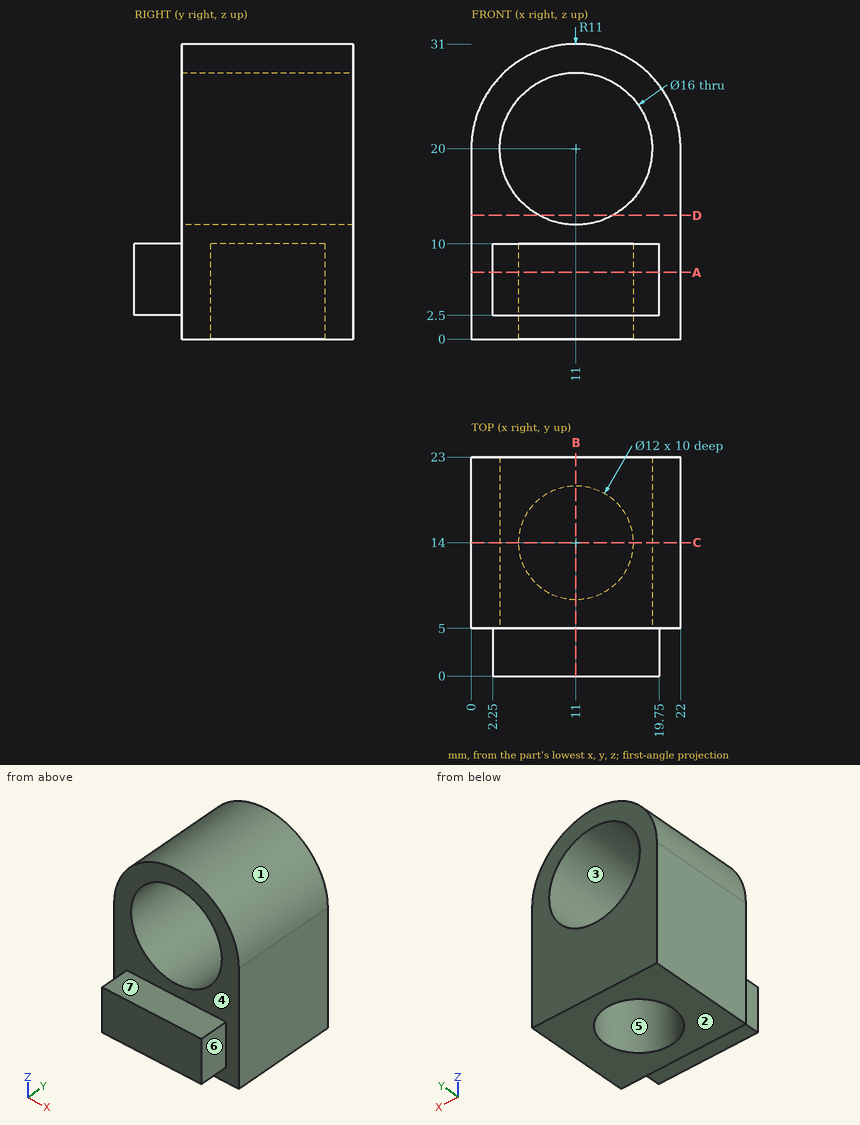
Input: dimensioned drawing with shaded views. Units: mm. Origin: part minimum x, y, z. A direction names the side the tool comes from. Coordinates: 2 decimals unless noted, no trailing zeros. Order: outer loops, then holes, each group sorted by start corner. A loop starts at its lowest first (then second) coordinate and runs counter-clockwise, first axis right, second up.
(1) Material intervals for probe 1 along Y at (x, z) = (11, 6.75); probe 2 along X at (y, z) = (17.75, 20); probe 3 along Z at (x, y) = (10, 2.5), sorted ascending.
(2) Section query C-C (y = 14). Return the cut outline in (x, z), plus the area to 3 significant figures.
(3) Draft query along Z for the marked faces 1, 2, 3 and 4. Return one class per face: pulls with the +Z half, pulls with the -Z half, needs draft (parallel to the pull), parting line crosses it, or undercut.
(4) Section query D-D (z = 13). Return the cut outline in (x, y).
(5) Access query for the marked faces 5, 6 and 7. Directions: +Z, -Z, +X, -X, +Y, -Y. A direction counts if a zero-diameter tool reaches every point of the face in a straight line with its end or side. Return the directions, or none.
(6) First-contact query: pin 1 (4 mm diameter, centred on x = 14, y = 2, fed in from -Z); pin 2 (2.5 mm diameter, centred on y = 2, z = 8, fed in from -X); pin 3 (1 mm diameter, centred on x = 19, y = 18.5, fed in from +Z). Flat tips, straight axial feed; report the tip coordinate or a pass-through.
(7) Section query A-A (z = 7). Return the cut outline in (x, y), plus the area to 3 significant figures.
(8) Section query B-B (x = 11). Return the cut outline in (y, z).
Solution:
1. probe 1: y = 0 to 8, 20 to 23
1. probe 2: x = 0 to 3, 19 to 22
1. probe 3: z = 2.5 to 10
2. outline: (0, 0) - (5, 0) - (5, 10) - (17, 10) - (17, 0) - (22, 0) - (22, 20) arc R11 ccw to (0, 20) - close; hole circle Ø16 at (11, 20)
2. area: 309 mm2
3. face 1: pulls with the +Z half
3. face 2: pulls with the -Z half
3. face 3: undercut
3. face 4: needs draft
4. outline: (0, 5) - (7.13, 5) - (7.13, 23) - (0, 23) - close; (14.87, 5) - (22, 5) - (22, 23) - (14.87, 23) - close
5. face 5: -Z
5. face 6: +Z, -Z, +X, -Y
5. face 7: +Z, +X, -X, -Y
6. pin 1: stops at z = 2.5
6. pin 2: stops at x = 2.25
6. pin 3: stops at z = 28.05
7. outline: (0, 5) - (2.25, 5) - (2.25, 0) - (19.75, 0) - (19.75, 5) - (22, 5) - (22, 23) - (0, 23) - close; hole circle Ø12 at (11, 14)
7. area: 370 mm2
8. outline: (0, 2.5) - (5, 2.5) - (5, 0) - (8, 0) - (8, 10) - (20, 10) - (20, 0) - (23, 0) - (23, 12) - (5, 12) - (5, 10) - (0, 10) - close; (5, 28) - (23, 28) - (23, 31) - (5, 31) - close
